from build123d import *

# Parameters (mm, degrees)
BOSS_EXTRUDE1_DEPTH = 58
SKETCH2_R           = 2
SKETCH2_R_2         = 20
CUT_EXTRUDE1_DEPTH  = 58
CUT_EXTRUDE2_DEPTH  = 58
CUT_EXTRUDE3_DEPTH  = 58
SKETCH5_R           = 2.95
BOSS_EXTRUDE2_DEPTH = 8
SKETCH6_R           = 3
SKETCH6_R_2         = 1.4
CUT_EXTRUDE4_DEPTH  = 8
SKETCH7_W           = 29
SKETCH7_H           = 6
CUT_EXTRUDE5_DEPTH  = 10


with BuildPart() as part:
    # Sketch1 → Boss-Extrude1 (new body)
    with BuildSketch(Plane(origin=(0, 0, 0), x_dir=(0, 0, -1), z_dir=(1, 0, 0))):
        Polygon((-73.351671883, 30.400809615), (-73.351671883, -29.599190385), (30.148328117, -29.599190385), (30.148328117, 30.400809615), (33.148328117, 30.400809615), (33.148328117, -32.599190385), (-76.351671883, -32.599190385), (-76.351671883, 30.400809615), align=None)
    extrude(amount=BOSS_EXTRUDE1_DEPTH)

    # Sketch2 → Cut-Extrude1 (cut)
    with BuildSketch(Plane.XY.offset(76.351671883)):
        with Locations((5.5, 24.900809615)):
            Circle(SKETCH2_R)
        with Locations((52.5, 24.900809615)):
            Circle(SKETCH2_R)
        with Locations((52.5, -22.099190385)):
            Circle(SKETCH2_R)
        with Locations((5.5, -22.099190385)):
            Circle(SKETCH2_R)
        with Locations((29, 1.400809615)):
            Circle(SKETCH2_R_2)
    extrude(amount=-CUT_EXTRUDE1_DEPTH, mode=Mode.SUBTRACT)

    # Sketch3 → Cut-Extrude2 (cut)
    with BuildSketch(Plane(origin=(0, 0, -33.148328117), x_dir=(-1, 0, 0), z_dir=(0, 0, -1))):
        with BuildLine():
            Line((-29, 30.400809615), (-58, 30.400809615))
            Line((-58, 30.400809615), (-58, 1.400809615))
            ThreePointArc((-58, 1.400809615), (-49.506096654, 21.90690627), (-29, 30.400809615))
        make_face()
    extrude(amount=-CUT_EXTRUDE2_DEPTH, mode=Mode.SUBTRACT)

    # Sketch4 → Cut-Extrude3 (cut)
    with BuildSketch(Plane(origin=(0, 0, -33.148328117), x_dir=(-1, 0, 0), z_dir=(0, 0, -1))):
        with BuildLine():
            Line((-29, 30.400809615), (0, 30.400809615))
            Line((0, 30.400809615), (0, 1.400809615))
            ThreePointArc((0, 1.400809615), (-8.493903346, 21.90690627), (-29, 30.400809615))
        make_face()
    extrude(amount=-CUT_EXTRUDE3_DEPTH, mode=Mode.SUBTRACT)

    # Sketch5 → Boss-Extrude2 (add)
    with BuildSketch(Plane(origin=(0, 0, -33.148328117), x_dir=(-1, 0, 0), z_dir=(0, 0, -1))):
        with Locations((-29, 1.400809615)):
            Circle(SKETCH5_R)
    extrude(amount=BOSS_EXTRUDE2_DEPTH)

    # Sketch6 → Cut-Extrude4 (cut)
    with BuildSketch(Plane.XZ.offset(32.599190385)):
        with Locations((29, 20.601671883)):
            Circle(SKETCH6_R)
        with Locations((29, 30.101671883)):
            Circle(SKETCH6_R_2)
        with Locations((37.227241336, 25.351671883)):
            Circle(SKETCH6_R_2)
        with Locations((37.227241336, 15.851671883)):
            Circle(SKETCH6_R_2)
        with Locations((29, 11.101671883)):
            Circle(SKETCH6_R_2)
        with Locations((20.772758664, 15.851671883)):
            Circle(SKETCH6_R_2)
        with Locations((20.772758664, 25.351671883)):
            Circle(SKETCH6_R_2)
    extrude(amount=-CUT_EXTRUDE4_DEPTH, mode=Mode.SUBTRACT)

    # Sketch7 → Cut-Extrude5 (cut)
    with BuildSketch(Plane.XY.offset(76.351671883)):
        with Locations((14.5, 1.400809615)):
            Rectangle(SKETCH7_W, SKETCH7_H)
    extrude(amount=-CUT_EXTRUDE5_DEPTH, mode=Mode.SUBTRACT)


solid = part.part
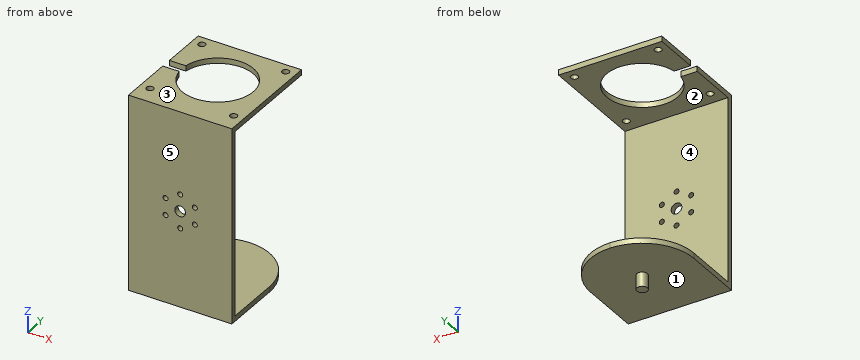
Could you check a few things on this model? Use its own coordinates, in mm. Face numbers are marked on the shaded views. A direction names the side the tool comes from. Give positions to 0.01 mm unless a question says otherwise; leave off trailing zeros. Order: outer loops, then holes, each group sorted by start corner. A loop starts at its lowest first (then second) coordinate and runs counter-clockwise, first axis right, second up. Notation, with made-up numbers: (67.25, 32) - (108.25, 32) arc R23 cw to (108.25, 49) - close; hole circle Ø1 at (18.25, -11.75). An arc over 180 degrees is marked (long way). Return JSON: item names as keys, results as strings. Group by question number.
Q1. Please list where these lines run through material, in increasing order: line 1 along Z through (x, y) = (29, -30.2); line 2 along Z through (x, y) = (53, 14.5); line 3 along Y through (x, z) = (29, 74.6). Write a range as [from, to].
Q2. Thinking about a two-plate mould opening in Z: for the marked faces 1, 2 and 3, which applies, pulls with the +Z half, pulls with the -Z half, needs draft (parallel to the pull), parting line crosses it, or undercut?
Q3. Suppose I cut it at B-B, the plane x = 52.5. Please give me the cut outline in (y, z), and give its area (3 significant figures).
Q4. Suppose I cut it at C-C, the plane x = 41. Please give me the cut outline in (y, z), and give its area (3 significant figures).
Q5. Will these pins go through, and if not, where does the flat tip stop? pin 1 Ø4.5 at (x, y) = (5.5, -22.1) entering from +Z; pin 2 Ø12 at (x, z) = (30.5, 21.5) entering from +Y; pin 3 Ø6 at (x, y) = (46, 14.5) entering from -Z; pin 4 Ø1.5 at (x, y) = (38, -7.5) entering from +Z.
Q6. Which directions (+Z, -Z, +X, -X, +Y, -Y) give clear straight access to the entire face, cutting with the end or side of a thin tool? Please do the marked faces 4 and 5.
Q7. Suppose I cut it at D-D, the plane y = -6.5. Please give me the cut outline in (x, z).
Q8. Suppose I cut it at A-A, the plane y = -28. Please give me the cut outline in (x, z).
Resolved:
{
 "1": {"line 1": "z = [-33.15, 9.7], [12.5, 17.6], [23.6, 28.7], [31.5, 76.35]", "line 2": "z = [-33.15, -30.15], [73.35, 76.35]", "line 3": "y = [-32.6, -18.6], [21.4, 30.4]"},
 "2": {"face 1": "pulls with the -Z half", "face 2": "undercut", "face 3": "pulls with the +Z half"},
 "3": {"outline": "(-32.6, -33.15) - (18.39, -33.15) - (18.39, -30.15) - (-29.6, -30.15) - (-29.6, 73.35) - (-24.1, 73.35) - (-24.1, 76.35) - (-32.6, 76.35) - close; (-20.1, 73.35) - (22.9, 73.35) - (22.9, 76.35) - (-20.1, 76.35) - close; (26.9, 73.35) - (30.4, 73.35) - (30.4, 76.35) - (26.9, 76.35) - close", "area": "628 mm2"},
 "4": {"outline": "(-32.6, -33.15) - (27.8, -33.15) - (27.8, -30.15) - (-29.6, -30.15) - (-29.6, 73.35) - (-14.6, 73.35) - (-14.6, 76.35) - (-32.6, 76.35) - close; (17.4, 73.35) - (30.4, 73.35) - (30.4, 76.35) - (17.4, 76.35) - close", "area": "585 mm2"},
 "5": {"pin 1": "stops at z = 76.35", "pin 2": "stops at y = -29.6", "pin 3": "stops at z = -33.15", "pin 4": "stops at z = -30.15"},
 "6": {"face 4": "+X, -X, +Y", "face 5": "+Z, -Z, +X, -X, -Y"},
 "7": {"outline": "(0, -33.15) - (58, -33.15) - (58, -30.15) - (0, -30.15) - close; (0, 73.35) - (10.63, 73.35) - (10.63, 76.35) - (0, 76.35) - close; (47.37, 73.35) - (58, 73.35) - (58, 76.35) - (47.37, 76.35) - close"},
 "8": {"outline": "(0, -33.15) - (58, -33.15) - (58, -30.15) - (0, -30.15) - close; (0, 73.35) - (58, 73.35) - (58, 76.35) - (0, 76.35) - close"}
}
